```python
from build123d import *

# Parameters (mm, degrees)
EXTRUDE_1_DEPTH     = 3
SKETCH_2_W          = 25
SKETCH_2_H          = 13
EXTRUDE_2_DEPTH     = 5
EXTRUDE_3_DEPTH     = 3
EXTRUDE_4_REACH     = 106.361
CUT_EXTRUDE_1_DEPTH = 105.987345913
SKETCH_6_W          = 6.056667596
SKETCH_6_H          = 33.940287548
CUT_EXTRUDE_2_DEPTH = 98.013364038
EXTRUDE_5_REACH     = 106.361
CUT_EXTRUDE_3_DEPTH = 3
CUT_EXTRUDE_4_DEPTH = 3
EXTRUDE_6_DEPTH     = 3
CUT_EXTRUDE_5_DEPTH = 105.633226751
SKETCH_12_R         = 5
CUT_EXTRUDE_6_DEPTH = 5
SKETCH_13_R         = 1.5
CUT_EXTRUDE_7_DEPTH = 5
SKETCH_14_R         = 1.5
CUT_EXTRUDE_8_DEPTH = 5
FILLET_1_DEPTH      = 3
FILLET_START        = 22
FILLET_1_2_DEPTH    = 3
FILLET_START_2      = 2.3595
FILLET_1_3_DEPTH    = 20


with BuildPart() as part:
    # 草图1 → 凸台-拉伸1 (new body)
    with BuildSketch(Plane.XY):
        Polygon((-98.335457187, 15.579868922), (-90.335457187, 15.579868922), (-90.335457187, 17.579868922), (-63.335457187, 4.579868922), (-61.335457187, 6.036256747), (-42.335457187, -2.420131078), (-39.335457187, -0.081665222), (-22.335457187, -6.420131078), (-10.835457187, -6.420131078), (5.664542813, -6.420131078), (5.664542813, -10.420131078), (-4.335457187, -19.420131078), (-6.381981311, -24.420131078), (-12.381981311, -24.420131078), (-13.29747583, -19.420131078), (-49.703887716, -10.420131078), (-79.703887716, -10.420131078), (-84.835457187, -14.420131078), (-90.835457187, -14.420131078), (-90.835457187, -7.719585483), (-98.335457187, 2.579868922), align=None)
    extrude(amount=EXTRUDE_1_DEPTH)

    # 草图2 → 凸台-拉伸2 (add)
    with BuildSketch(Plane.ZY.offset(98.335457187)):
        with Locations((12.5, 9.079868922)):
            Rectangle(SKETCH_2_W, SKETCH_2_H)
    extrude(amount=-EXTRUDE_2_DEPTH)

    # 草图3 → 凸台-拉伸3 (add)
    with BuildSketch(Plane.XY.offset(25)):
        Polygon((-90.335457187, 15.579868922), (-98.335457187, 15.579868922), (-98.335457187, 2.579868922), (-90.835457187, -7.719585483), (-90.835457187, -14.420131078), (-84.835457187, -14.420131078), (-79.703887716, -10.420131078), (-49.703887716, -10.420131078), (-13.29747583, -19.420131078), (-12.381981311, -24.420131078), (-6.381981311, -24.420131078), (-4.335457187, -19.420131078), (5.664542813, -10.420131078), (5.664542813, -6.420131078), (-22.335457187, -6.420131078), (-39.335457187, -0.081665222), (-42.335457187, -2.420131078), (-61.335457187, 6.036256747), (-63.335457187, 4.579868922), (-90.335457187, 17.579868922), align=None)
    extrude(amount=-EXTRUDE_3_DEPTH)

    # 草图4 → 凸台-拉伸4 (add, up to next)
    with BuildSketch(Plane.XY.offset(25), mode=Mode.PRIVATE) as extrude_4_sk1:
        Polygon((-98.335457187, 2.579868922), (-90.835457187, -7.719585483), (-90.835457187, -14.420131078), (-84.835457187, -14.420131078), (-84.835457187, -9.420131078), (-85.835457187, -9.420131078), (-85.835457187, -6.09200144), (-92.150260395, 2.579868922), align=None)
    extrude_4_tool1 = extrude(extrude_4_sk1.sketch, amount=-EXTRUDE_4_REACH, mode=Mode.PRIVATE) - part.part
    add(extrude_4_tool1.solids().sort_by_distance((-90.201592, -5.80053, 25))[0])

    # 草图5 → 切除-拉伸1 (cut, through all)
    with BuildSketch(Plane(origin=(-93.335457187, 0, 0), x_dir=(0, 0, -1), z_dir=(1, 0, 0))):
        with BuildLine():
            Line((-16.657130076, 15.579868922), (-8.342869924, 15.579868922))
            ThreePointArc((-8.342869924, 15.579868922), (-9.779019247, 10.678144674), (-12.5, 6.355450003))
            ThreePointArc((-12.5, 6.355450003), (-15.220980753, 10.678144674), (-16.657130076, 15.579868922))
        make_face()
    extrude(amount=-CUT_EXTRUDE_1_DEPTH, mode=Mode.SUBTRACT)

    # 草图6 → 切除-拉伸2 (cut, through all)
    with BuildSketch(Plane(origin=(-84.835457187, 0, 0), x_dir=(0, 0, -1), z_dir=(1, 0, 0))):
        with Locations((-12.5, -14.420131078)):
            Rectangle(SKETCH_6_W, SKETCH_6_H)
    extrude(amount=-CUT_EXTRUDE_2_DEPTH, mode=Mode.SUBTRACT)

    # 草图7 → 凸台-拉伸5 (add, up to next)
    with BuildSketch(Plane(origin=(0, 0, 0), x_dir=(-1, 0, 0), z_dir=(0, 0, -1)), mode=Mode.PRIVATE) as extrude_5_sk1:
        Polygon((41.335457187, -1.64064246), (39.335457187, -0.081665222), (39.335457187, -12.983302507), (41.335457187, -12.488884104), align=None)
    extrude_5_tool1 = extrude(extrude_5_sk1.sketch, amount=-EXTRUDE_5_REACH, mode=Mode.PRIVATE) - part.part
    # 草图7 → 凸台-拉伸5 (add, up to next)
    with BuildSketch(Plane(origin=(0, 0, 0), x_dir=(-1, 0, 0), z_dir=(0, 0, -1)), mode=Mode.PRIVATE) as extrude_5_sk2:
        Polygon((59.961995831, 5.424966121), (59.961995831, -10.420131078), (61.961995831, -10.420131078), (61.961995831, 5.580015121), (61.335457187, 6.036256747), align=None)
    extrude_5_tool2 = extrude(extrude_5_sk2.sketch, amount=-EXTRUDE_5_REACH, mode=Mode.PRIVATE) - part.part
    add(extrude_5_tool1.solids().sort_by_distance((-40.306637, -6.790953, 0))[0])
    add(extrude_5_tool2.solids().sort_by_distance((-60.965536, -2.331748, 0))[0])

    # 草图8 → 切除-拉伸3 (cut)
    with BuildSketch(Plane(origin=(-39.335457187, 0, 0), x_dir=(0, 0, -1), z_dir=(1, 0, 0))):
        with BuildLine():
            Line((-20.2471791, -12.983302507), (-4.7528209, -12.983302507))
            ThreePointArc((-4.7528209, -12.983302507), (-12.5, -4.669641244), (-20.2471791, -12.983302507))
        make_face()
    extrude(amount=-CUT_EXTRUDE_3_DEPTH, mode=Mode.SUBTRACT)

    # 草图9 → 切除-拉伸4 (cut)
    with BuildSketch(Plane(origin=(-59.961995831, 0, 0), x_dir=(0, 0, -1), z_dir=(1, 0, 0))):
        with BuildLine():
            Line((-20.000265411, -10.420131078), (-4.999734589, -10.420131078))
            ThreePointArc((-4.999734589, -10.420131078), (-12.5, -2.919865667), (-20.000265411, -10.420131078))
        make_face()
    extrude(amount=-CUT_EXTRUDE_4_DEPTH, mode=Mode.SUBTRACT)

    # 草图10 → 凸台-拉伸6 (add)
    with BuildSketch(Plane(origin=(0, -6.420131078, 0), x_dir=(1, 0, 0), z_dir=(0, 1, 0))):
        with BuildLine():
            Line((-26.085728059, -3), (-26.085728059, 0))
            Line((-26.085728059, 0), (-14.640217294, 0))
            ThreePointArc((-14.640217294, 0), (5.664542813, -12.5), (-14.640217294, -25))
            Line((-14.640217294, -25), (-26.085728059, -25))
            Line((-26.085728059, -25), (-26.085728059, -22))
            ThreePointArc((-26.085728059, -22), (-23.536750664, -12.5), (-26.085728059, -3))
        make_face()
    extrude(amount=-EXTRUDE_6_DEPTH)

    # 草图11 → 切除-拉伸5 (cut, through all)
    with BuildSketch(Plane(origin=(0, -6.420131078, 0), x_dir=(1, 0, 0), z_dir=(0, 1, 0))):
        with BuildLine():
            Line((-2.030697081, 0), (16.123773985, 18.747228403))
            Line((16.123773985, 18.747228403), (16.123773985, -39.39165183))
            Line((16.123773985, -39.39165183), (-2.030697081, -25))
            ThreePointArc((-2.030697081, -25), (5.664542813, -12.5), (-2.030697081, 0))
        make_face()
    extrude(amount=-CUT_EXTRUDE_5_DEPTH, mode=Mode.SUBTRACT)

    # 草图12 → 切除-拉伸6 (cut)
    with BuildSketch(Plane(origin=(0, -6.420131078, 0), x_dir=(1, 0, 0), z_dir=(0, 1, 0))):
        with Locations(Location((-8.335457187, -12.5, 0), (0, 0, 180))):
            Circle(SKETCH_12_R)
        with BuildLine():
            Line((-1.527591385, -17.186545459), (0.125093583, -18.839230427))
            ThreePointArc((0.125093583, -18.839230427), (0.125093583, -20.960550771), (-1.99622676, -20.960550771))
            Line((-1.99622676, -20.960550771), (-3.648911729, -19.307865802))
            ThreePointArc((-3.648911729, -19.307865802), (-3.648911729, -17.186545459), (-1.527591385, -17.186545459))
        make_face()
        with BuildLine():
            Line((-13.022002646, -19.307865802), (-14.674687614, -20.960550771))
            ThreePointArc((-14.674687614, -20.960550771), (-16.796007958, -20.960550771), (-16.796007958, -18.839230427))
            Line((-16.796007958, -18.839230427), (-15.143322989, -17.186545459))
            ThreePointArc((-15.143322989, -17.186545459), (-13.022002646, -17.186545459), (-13.022002646, -19.307865802))
        make_face()
        with BuildLine():
            Line((-15.143322989, -7.813454541), (-16.796007958, -6.160769573))
            ThreePointArc((-16.796007958, -6.160769573), (-16.796007958, -4.039449229), (-14.674687614, -4.039449229))
            Line((-14.674687614, -4.039449229), (-13.022002646, -5.692134198))
            ThreePointArc((-13.022002646, -5.692134198), (-13.022002646, -7.813454541), (-15.143322989, -7.813454541))
        make_face()
        with BuildLine():
            Line((-3.648911729, -5.692134198), (-1.99622676, -4.039449229))
            ThreePointArc((-1.99622676, -4.039449229), (0.125093583, -4.039449229), (0.125093583, -6.160769573))
            Line((0.125093583, -6.160769573), (-1.527591385, -7.813454541))
            ThreePointArc((-1.527591385, -7.813454541), (-3.648911729, -7.813454541), (-3.648911729, -5.692134198))
        make_face()
    extrude(amount=-CUT_EXTRUDE_6_DEPTH, mode=Mode.SUBTRACT)

    # 草图13 → 切除-拉伸7 (cut)
    with BuildSketch(Plane(origin=(0, 15.579868922, 0), x_dir=(1, 0, 0), z_dir=(0, 1, 0))):
        with Locations(Location((-95.835457187, -5, 0), (0, 0, 270))):
            Circle(SKETCH_13_R)
        with Locations(Location((-95.835457187, -20, 0), (0, 0, 270))):
            Circle(SKETCH_13_R)
    extrude(amount=-CUT_EXTRUDE_7_DEPTH, mode=Mode.SUBTRACT)

    # 草图14 → 切除-拉伸8 (cut)
    with BuildSketch(Plane.XZ.offset(14.420131078)):
        with Locations(Location((-88.335457187, 20, 0), (0, 0, 270))):
            Circle(SKETCH_14_R)
        with Locations(Location((-88.335457187, 5, 0), (0, 0, 270))):
            Circle(SKETCH_14_R)
    extrude(amount=-CUT_EXTRUDE_8_DEPTH, mode=Mode.SUBTRACT)

    # 圆角1: read off the stored shape, not the designer's step
    # 圆角1 outline → 圆角1 (add)
    with BuildSketch(Plane.XY):
        with BuildLine():
            ThreePointArc((-39.969314292, -0.575749621), (-42.436321647, -1.595291169), (-45.076309168, -1.200251746))
            Line((-45.076309168, -1.200251746), (-42.335457187, -2.420131078))
            Line((-42.335457187, -2.420131078), (-39.969314292, -0.575749621))
        make_face()
        with BuildLine():
            ThreePointArc((-61.335457187, 6.036256747), (-63.646870744, 5.371779089), (-66.001128729, 5.863340405))
            Line((-66.001128729, 5.863340405), (-63.335457187, 4.579868922))
            Line((-63.335457187, 4.579868922), (-61.335457187, 6.036256747))
        make_face()
    extrude(amount=FILLET_1_DEPTH)

    # Fillet 1 2 outline → Fillet 1 2 (add)
    with BuildSketch(Plane.XY.offset(FILLET_START)):
        with BuildLine():
            ThreePointArc((-39.969314292, -0.575749621), (-42.436321647, -1.595291169), (-45.076309168, -1.200251746))
            Line((-45.076309168, -1.200251746), (-42.335457187, -2.420131078))
            Line((-42.335457187, -2.420131078), (-39.969314292, -0.575749621))
        make_face()
        with BuildLine():
            ThreePointArc((-61.335457187, 6.036256747), (-63.646870744, 5.371779089), (-66.001128729, 5.863340405))
            Line((-66.001128729, 5.863340405), (-63.335457187, 4.579868922))
            Line((-63.335457187, 4.579868922), (-61.335457187, 6.036256747))
        make_face()
    extrude(amount=FILLET_1_2_DEPTH)

    # Fillet 1 3 outline → Fillet 1 3 (add)
    with BuildSketch(Plane.XY.offset(FILLET_START_2)):
        with BuildLine():
            Line((-41.335457187, -1.64064246), (-39.969314292, -0.575749621))
            ThreePointArc((-39.969314292, -0.575749621), (-40.622702266, -1.007314283), (-41.335457187, -1.331573939))
            Line((-41.335457187, -1.331573939), (-41.335457187, -1.64064246))
        make_face()
        with BuildLine():
            Line((-61.961995831, 5.580015121), (-61.335457187, 6.036256747))
            ThreePointArc((-61.335457187, 6.036256747), (-61.643406083, 5.872813744), (-61.961995831, 5.731227337))
            Line((-61.961995831, 5.731227337), (-61.961995831, 5.580015121))
        make_face()
    extrude(amount=FILLET_1_3_DEPTH)


solid = part.part
```
Geometry: final body of the model. Coordinates: model frame, mm. A direction names the side the tool comes from. Round coordinates to 2 decimals unless told otherwise and drop trailing zeros. Write each loop counter-clockwise with the first axis right and the second up, starting at its lowest first coordinate (ties: lowest second). Pieces come first, ordered by that corner, then holes.
Item 1: Material intervals for L1, parallel to Z at x = -94, y = -1; L2, parallel to X at y = -10.75, z = 20; L3, parallel to X at y = -9, z = 5.75, sorted ascending.
Item 2: Section query C-C (z = 23.5). Return loops of the section in (x, y).
Item 3: Section query A-A (y = -21). Return loops of the section in (x, z), plus the area to 3 significant figures.
Item 4: Set-up query: faces 1 (the face through (-41.335, -4, 12)), 2 (the face through (-89.666, -11.955, 4.308)), 3 (the face through (-96, 10.58, 5)). Return all of +Z, -Z, +X, -X, +Y, -Y with unobstructed straight access to the full face (end or side cutting, diameter ignored); none if empty.
Item 5: Mould query, pull axis Z, two halves, no side actions, for faces 4 (the face through (-95, -2, 7)), 5 (the face through (-90, -6, 15.528)), 6 (the face through (-95.8, 10.74, 9.75)). Classes: +Z half, -Z half, draft (parallel to the pull), parting line (faces both ways), or undercut.
Item 6: Section query D-D (x = -20). Return loops of the section in (y, z), plus the area to 3 significant figures.
Item 7: Section query B-B (x = -54). Return loops of the section in (y, z).
Item 8: Pin query (flat end, axial travel): P1, Ø6, axis at x = -12.5, z = 17, coming from the +Y side; P2, Ø2.5, axis at x = -94.5, z = 3, coming from the +Y side; P3, Ø2.5, axis at x = -96, z = 5, coming from the +Y side. Return the tip coordinate at first contact, or that it passes through.
Completed:
1. L1: z = 0 to 9.47, 15.53 to 25
1. L2: x = -90.84 to -89.84, -86.84 to -84.84
1. L3: x = -90.84 to -85.84, -24.78 to -17.09, -12.97 to -3.7, 0.42 to 3.93
2. outline: (-98.34, 2.58) - (-90.84, -7.72) - (-90.84, -14.42) - (-84.84, -14.42) - (-79.7, -10.42) - (-49.7, -10.42) - (-13.3, -19.42) - (-12.38, -24.42) - (-6.38, -24.42) - (-4.34, -19.42) - (0.32, -15.23) - (0.32, -6.42) - (-22.34, -6.42) - (-39.34, -0.08) - (-39.97, -0.58) arc R5 cw to (-45.08, -1.2) - (-61.34, 6.04) arc R5 cw to (-66, 5.86) - (-90.34, 17.58) - (-90.34, 15.58) - (-98.34, 15.58) - close
3. outline: (-13.01, 0) - (-4.98, 0) - (-4.98, 3) - (-13.01, 3) - close; (-13.01, 22) - (-4.98, 22) - (-4.98, 25) - (-13.01, 25) - close
3. area: 48.2 mm2
4. face 1: +Y, -Y
4. face 2: -Y
4. face 3: +Y
5. face 4: draft
5. face 5: undercut
5. face 6: undercut
6. outline: (-17.76, 0) - (-6.42, 0) - (-6.42, 25) - (-17.76, 25) - (-17.76, 22) - (-9.42, 22) - (-9.42, 3) - (-17.76, 3) - close
6. area: 125 mm2
7. outline: (-10.42, 0) - (2.77, 0) - (2.77, 3) - (-10.42, 3) - close; (-10.42, 22) - (2.77, 22) - (2.77, 25) - (-10.42, 25) - close
8. P1: stops at y = -6.42
8. P2: stops at y = 15.58
8. P3: stops at y = 10.58
